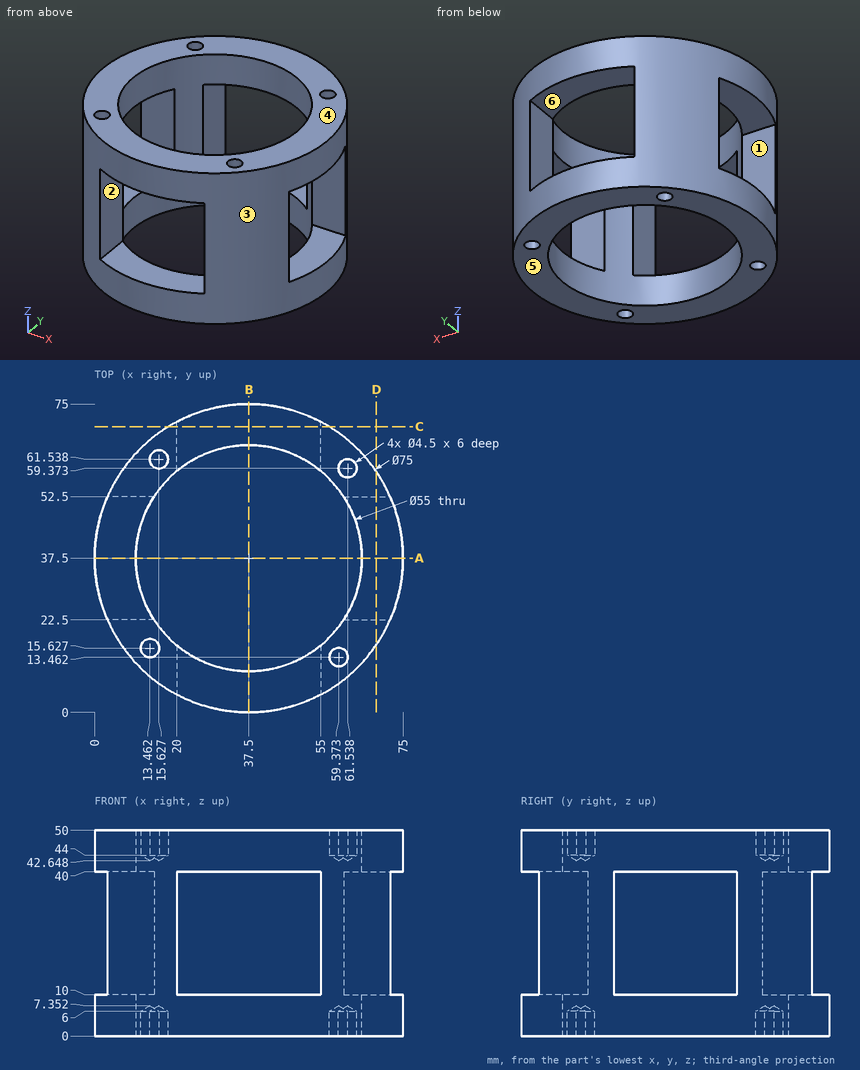
The drawing under review shows one solid part. Ordinate dimensions are in mm from its lowest x, y, z. A direction names the side the tool comes from. Round coordinates to 2 decimals unless told otherwise and drop trailing zeros. Write each loop counter-clockwise with the first axis right and the second up, starting at its lowest first coordinate (ties: lowest second). Pieces come first, ordered by that corner, then holes. Notation, with made-up numbers: (-19.75, 57) -> (24.25, 57) arc R30 ccw to (24.25, 79) -> close; hole circle Ø1 at (76.5, 74.25). An arc over 180 degrees is marked (long way). One line per question, with ' | ' between items. Start each with the question number.
(1) Add section A-A, the plane y = 37.5. Write out the cut boundary in (x, z).
(2) Add section D-D, the plane x = 68.5. Write out the cut boundary in (y, z).
(3) Tool access review of the marked faces 1, 2 and 3: name each direction out of +Z, -Z, +X, -X, +Y, -Y from which nothing blocks a thin tool from reaching the whole face with its end or side.
(4) For line 1 along X through (y, z) = (20, 44); line 2 along Y through (x, z) = (52, 4); line 3 along X through (y, z) = (53, 25) (1 decimal), list the stretches that pass through material, from the lowest coordinate up. Write a range as from..to.
(5) Add section C-C, the plane y = 69.5. Write out the cut boundary in (x, z), plus the area to 3 significant figures.
(6) Mouldability with a two-part tool opening along Z and no side actions: class the marked faces 4, 5 and 6 as released by +Z, released by -Z, zero draft, split by the parting line, or undercut.
(7) Insertion check: P1, Ø3.5, axis at y = 9, z = 30.5, coming from the -X side; P2, Ø6, axis at y = 62.5, z = 25.5, coming from the -X side; P3, Ø3, axis at x = 19, z = 30, coming from the +Y side. Each pin has a flat end and moves straight along its axis. Give the tip position at first contact, or say it passes through.
Answer list:
1) outline: (0, 0) -> (10, 0) -> (10, 10) -> (0, 10) -> close; (0, 40) -> (10, 40) -> (10, 50) -> (0, 50) -> close; (65, 0) -> (75, 0) -> (75, 10) -> (65, 10) -> close; (65, 40) -> (75, 40) -> (75, 50) -> (65, 50) -> close
2) outline: (16.4, 0) -> (58.6, 0) -> (58.6, 50) -> (16.4, 50) -> close; hole (22.5, 10) -> (52.5, 10) -> (52.5, 40) -> (22.5, 40) -> close
3) face 1: +X, -X | face 2: +Y, -Y | face 3: +Z, -Z
4) line 1: 4.33..16.29, 58.71..70.67 | line 2: 2.92..14.13, 60.87..72.08 | line 3: 3.4..14.8, 60.2..71.6
5) outline: (17.95, 0) -> (57.05, 0) -> (57.05, 50) -> (17.95, 50) -> close; hole (20, 10) -> (55, 10) -> (55, 40) -> (20, 40) -> close | area: 905 mm²
6) face 4: released by +Z | face 5: released by -Z | face 6: undercut
7) P1: x = 11.22 | P2: x = 7.13 | P3: y = 70.67
